```python
from build123d import *

# Parameters (mm, degrees)
SKETCH1_R           = 0.605786837
BOSS_EXTRUDE1_DEPTH = 10
SKETCH3_R           = 30
SKETCH3_R_2         = 15
CUT_EXTRUDE1_DEPTH  = 10


with BuildPart() as part:
    # Sketch1 → Boss-Extrude1 (new body)
    with BuildSketch(Plane(origin=(0, 0, 0), x_dir=(1, 0, 0), z_dir=(0, 1, 0))):
        with BuildLine():
            Line((42.395388783, 14.504200511), (45.014187909, 17.812893064))
            ThreePointArc((45.014187909, 17.812893064), (95.299132477, -4.289618646), (45.014187909, -26.392130356))
            Line((45.014187909, -26.392130356), (42.395388783, -23.083437803))
            ThreePointArc((42.395388783, -23.083437803), (38.909611349, -20.287901909), (34.554258804, -19.289618646))
            Line((34.554258804, -19.289618646), (-90.607383501, -19.289618646))
            ThreePointArc((-90.607383501, -19.289618646), (-94.579180908, -20.112210224), (-97.897544897, -22.444653576))
            Line((-97.897544897, -22.444653576), (-105.310368622, -30.339607137))
            ThreePointArc((-105.310368622, -30.339607137), (-163.685528507, -4.289618646), (-105.310368622, 21.760369845))
            Line((-105.310368622, 21.760369845), (-97.897544897, 13.865416283))
            ThreePointArc((-97.897544897, 13.865416283), (-94.579180908, 11.532972931), (-90.607383501, 10.710381354))
            Line((-90.607383501, 10.710381354), (34.554258804, 10.710381354))
            ThreePointArc((34.554258804, 10.710381354), (38.909611349, 11.708664617), (42.395388783, 14.504200511))
        make_face()
        with Locations(Location((65.299132477, -4.289618646, 0), (0, 0, 270))):
            Circle(SKETCH1_R, mode=Mode.SUBTRACT)
    extrude(amount=BOSS_EXTRUDE1_DEPTH)

    # Sketch3 → Cut-Extrude1 (cut)
    with BuildSketch(Plane(origin=(0, 10, 0), x_dir=(1, 0, 0), z_dir=(0, 1, 0))):
        with Locations(Location((-128.685528507, -4.289618646, 0), (0, 0, 270))):
            Circle(SKETCH3_R)
        with Locations(Location((65.664200703, -4.773046906, 0), (0, 0, 270))):
            Circle(SKETCH3_R_2)
    extrude(amount=-CUT_EXTRUDE1_DEPTH, mode=Mode.SUBTRACT)


solid = part.part
```
CAD build for the part. Positions are in the model's coordinates, mm. A direction names the side the tool comes from. Coordinates: 2 decimals unless noted, no trailing zeros. Order: outer loops, then holes, each group sorted by start corner. A loop starts at its lowest first (then second) coordinate and runs counter-clockwise, first axis right, second up.
(1) Saw through at C-C, the plane z = 0.5. Write the cut outline in (x, y).
Solution:
outline: (-163.48, 0) - (-158.45, 0) - (-158.45, 10) - (-163.48, 10) - close; (-98.93, 0) - (51.29, 0) - (51.29, 10) - (-98.93, 10) - close; (80.04, 0) - (95.06, 0) - (95.06, 10) - (80.04, 10) - close
(2) Which spindle directions (+Z, -Z, +X, -X, +Y, -Y) get a long thin tool onto all of the face, cutting with end or side? Do faces 5 (the face through (38.85, 4.93, -11.68)), 6 (the face through (-27, 5, 19.29)), 7 (the face through (-14, 10, 4)). Say none if no direction does.
Solution:
face 5: -Z, +Y, -Y
face 6: +Z, +Y, -Y
face 7: +Z, -Z, +X, -X, +Y
(3) Drill centre lines: L1, parallel to X at y = 5, z = -16.5; L2, parallel to X at y = 1.5, z = -4.5; L3, parallel to Z at x = -73, y = 5.75. Where is each one in solid material? Low to high.
Solution:
L1: x = -156.84 to -150.31, -107.06 to -100.37, 43.98 to 86.93
L2: x = -162.56 to -157.37, -100 to 53.87, 77.45 to 93.98
L3: z = -10.71 to 19.29
(4) Pin check, flat tips, straight feed: pin 1 Ø6 at (y, z) = (1, -2) entering from +X; pin 2 Ø5 at (x, y) = (-21, 4.5) entering from -Z; pin 3 Ø5 at (x, y) = (-46.5, 4) entering from +Z; pin 4 Ø4 at (x, z) = (40.5, 25) entering from -Y. Stop position of each tip, or through.
Solution:
pin 1: stops at x = 95.12
pin 2: stops at z = -10.71
pin 3: stops at z = 19.29
pin 4: passes through
(5) Saw through at B-B, the plane y = 5.5. Write the cut outline in (x, z), and give its area (3 significant figures).
Solution:
outline: (-105.31, -21.76) - (-97.9, -13.87) arc R10 cw to (-90.61, -10.71) - (34.55, -10.71) arc R10 cw to (42.4, -14.5) - (45.01, -17.81) arc R30 ccw (long way) to (45.01, 26.39) - (42.4, 23.08) arc R10 cw to (34.55, 19.29) - (-90.61, 19.29) arc R10 cw to (-97.9, 22.44) - (-105.31, 30.34) arc R35 ccw (long way) to start; hole circle Ø60 at (-128.69, 4.29); hole circle Ø30 at (65.66, 4.77)
area: 7,100 mm2
(6) Mould opens along Z. For faces 1 (the face through (-101.66, 4.93, -17.87)), 2 (the face through (95.283, 4.93, 3.318)), 3 (the face through (38.966, 4.93, 20.316)), 4 (the face through (51.02, 5.07, 1.52)) say: released by +Z, released by -Z, zero draft, split by the parting line, or undercut.
Solution:
face 1: released by -Z
face 2: split by the parting line
face 3: released by +Z
face 4: undercut
(7) Saw through at A-A, the plane z = 15.5. Write the cut outline in (x, y), and give its area (3 significant figures).
Solution:
outline: (-161.84, 0) - (-156.51, 0) - (-156.51, 10) - (-161.84, 10) - close; (-100.86, 0) - (55.18, 0) - (55.18, 10) - (-100.86, 10) - close; (76.15, 0) - (93.13, 0) - (93.13, 10) - (76.15, 10) - close
area: 1,780 mm2
(8) Saw through at D-D, the plane x = -12. Write the cut outline in (y, z).
Solution:
outline: (0, -10.71) - (10, -10.71) - (10, 19.29) - (0, 19.29) - close
